Here's how the part is built. I have some questions about the finished solid (model axes, mm). A direction names the side the tool comes from. Give positions to 0.01 mm unless a question says otherwise; leave off trailing zeros. Order: outer loops, then holes, each group sorted by start corner. A loop starts at its lowest first (then second) coordinate and runs counter-clockwise, first axis right, second up.
from build123d import *

# Parameters (mm, degrees)
F1_DEPTH = 12.7
F2_R     = 1.25
F2_R_2   = 1.55
F3_DEPTH = 6


with BuildPart() as f1:
    # F0 (on Front) → F1 (new body)
    with BuildSketch(Plane.XZ):
        with BuildLine():
            ThreePointArc((10.472688, 2.032), (0, -10.668), (-10.472688, 2.032))
            Line((-10.472688, 2.032), (-14.142264, 2.032))
            ThreePointArc((-14.142264, 2.032), (-14.251145, 1.018592), (-14.2875, 0))
            Line((-14.2875, 0), (-14.2875, -13.843))
            Line((-14.2875, -13.843), (14.2875, -13.843))
            Line((14.2875, -13.843), (14.2875, 0))
            ThreePointArc((14.2875, 0), (14.251145, 1.018592), (14.142264, 2.032))
            Line((14.142264, 2.032), (10.472688, 2.032))
        make_face()
    extrude(amount=F1_DEPTH)

    # F2 (on face) → F3 (cut)
    with BuildSketch(Plane(origin=(0, 0, -13.843), x_dir=(1, 0, 0), z_dir=(0, 0, -1))):
        with Locations((-11, 6.35)):
            Circle(F2_R)
        with Locations((11, 6.35)):
            Circle(F2_R)
        with Locations((0, 6.35)):
            Circle(F2_R_2)
    extrude(amount=-F3_DEPTH, mode=Mode.SUBTRACT)


solid = f1.part
Q1. If we section it at A-A on y = -6.35: List the corners of the cut face in (x, z) for me.
Filled sheet:
outline: (-14.29, -13.84) - (-12.25, -13.84) - (-12.25, -7.84) - (-9.75, -7.84) - (-9.75, -13.84) - (-1.55, -13.84) - (-1.55, -10.55) arc R10.67 cw to (-10.47, 2.03) - (-14.14, 2.03) arc R14.29 ccw to (-14.29, 0) - close; (1.55, -13.84) - (9.75, -13.84) - (9.75, -7.84) - (12.25, -7.84) - (12.25, -13.84) - (14.29, -13.84) - (14.29, 0) arc R14.29 ccw to (14.14, 2.03) - (10.47, 2.03) arc R10.67 cw to (1.55, -10.55) - close
Q2. I need wall thicknesses on L1, parallel to X at y = -6.35, z = -12.35; L2, parallel to X at y = -3.75, z = 0; L3, parallel to Y at x = 0, z = -12.4. Which ranges of each line are inside material? Lowest first, please.
Filled sheet:
L1: x = -14.29 to -12.25, -9.75 to -1.55, 1.55 to 9.75, 12.25 to 14.29
L2: x = -14.29 to -10.67, 10.67 to 14.29
L3: y = -12.7 to -7.9, -4.8 to 0
Q3. I'm going to push flat-ended pins straight in: P1, Ø1.2, axis at x = 10.5, y = -6, coming from the -Z side; P2, Ø1, axis at x = -6, z = -8.5, coming from the +Y side. Where does each tip first touch, or does it pass through?
Filled sheet:
P1: stops at z = -7.84
P2: stops at y = 0
Q4. Thinking about a two-plate mould opening in Y: for faces 3 (the face through (0.715, -4.975, -12.22)), 4 (the face through (14.252, -6.261, 1.004)), 5 (the face through (0, -12.7, -11)), which applies, released by +Y, released by -Y, zero draft, split by the parting line, or undercut?
Filled sheet:
face 3: undercut
face 4: zero draft
face 5: released by -Y
Q5. If we section it at B-B on x = 0: List the corners of the cut face in (y, z) for me, plus the area to 3 significant figures.
Filled sheet:
outline: (-12.7, -13.84) - (-7.9, -13.84) - (-7.9, -10.67) - (-12.7, -10.67) - close; (-4.8, -13.84) - (0, -13.84) - (0, -10.67) - (-4.8, -10.67) - close
area: 30.5 mm2
Q6. If we section it at C-C on z = -9.5: List the corners of the cut face in (x, y) for me, plus the area to 3 significant figures.
Filled sheet:
outline: (-14.29, -12.7) - (-4.85, -12.7) - (-4.85, 0) - (-14.29, 0) - close; (4.85, -12.7) - (14.29, -12.7) - (14.29, 0) - (4.85, 0) - close; hole circle Ø2.5 at (-11, -6.35); hole circle Ø2.5 at (11, -6.35)
area: 230 mm2
Q7. For faces 1 (the face through (-12.25, -6.4, -10.88)), 2 (the face through (12, -6, 2.032)), which set-ups out of +Z, -Z, +X, -X, +Y, -Y let a thin tool reach every point of the face, with its end or its side?
Filled sheet:
face 1: -Z
face 2: +Z, +X, -X, +Y, -Y
Q8. If we section it at D-D on y = -3: List the corners of the cut face in (x, z) for me, plus the area to 3 significant figures.
Filled sheet:
outline: (-14.29, -13.84) - (14.29, -13.84) - (14.29, 0) arc R14.29 ccw to (14.14, 2.03) - (10.47, 2.03) arc R10.67 cw (long way) to (-10.47, 2.03) - (-14.14, 2.03) arc R14.29 ccw to (-14.29, 0) - close
area: 232 mm2
